Read the model definition and answer for the solid it produces. Units are mm, in the model's axes. A direction names the side the tool comes from. Give positions to 0.01 mm unless a question says otherwise; leave off trailing zeros. Loops run counter-clockwise (first coordinate to the right, second up) from the corner with the lowest first, then second, coordinate; pieces in that order, holes last. Notation, with made-up numbers: (48, 46.5) - (69, 46.5) arc R14 ccw to (69, 54.5) - close; hole circle Ø2 at (-29, 71.5). An arc over 180 degrees is marked (long way). Write item = value, one per line.
```python
from build123d import *

# Parameters (mm, degrees)
BOSS_EXTRUDE1_DEPTH = 1.524


with BuildPart() as part:
    # Sketch1 → Boss-Extrude1 (new body)
    with BuildSketch(Plane.XY):
        with BuildLine():
            Line((25.899875794, 0), (25.899875794, -1.524))
            Line((25.899875794, -1.524), (22.32048354, -1.524))
            ThreePointArc((22.32048354, -1.524), (22.394704152, -2.448389179), (22.608367924, -3.350803633))
            ThreePointArc((22.608367924, -3.350803633), (24.775682693, -15.358642742), (23.925034543, -27.530818024))
            ThreePointArc((23.925034543, -27.530818024), (24.269313487, -29.941018013), (26.694765546, -30.152617376))
            ThreePointArc((26.694765546, -30.152617376), (43.800025443, -37.203050355), (61.874254559, -41.155361478))
            ThreePointArc((61.874254559, -41.155361478), (63.35881503, -45.79590736), (63.615238945, -50.661380887))
            ThreePointArc((63.615238945, -50.661380887), (65.284550388, -52.552507853), (66.8346767, -50.562515312))
            ThreePointArc((66.8346767, -50.562515312), (66.086863923, -45.883082095), (65.762862434, -41.155361478))
            ThreePointArc((65.762862434, -41.155361478), (66.787088001, -38.530646728), (65.033651376, -36.325283826))
            ThreePointArc((65.033651376, -36.325283826), (63.508505747, -35.385780492), (62.493571354, -33.909757498))
            ThreePointArc((62.493571354, -33.909757498), (60.142882659, -34.378985159), (58.743656643, -36.325283826))
            ThreePointArc((58.743656643, -36.325283826), (57.410289813, -36.601347141), (56.250770366, -35.887489516))
            ThreePointArc((56.250770366, -35.887489516), (55.059942052, -35.328446838), (53.862175702, -34.784427942))
            ThreePointArc((53.862175702, -34.784427942), (53.387744375, -32.845536507), (52.235990682, -31.215245578))
            ThreePointArc((52.235990682, -31.215245578), (52.379437809, -32.619080701), (52.025456966, -33.985106943))
            ThreePointArc((52.025456966, -33.985106943), (49.256787636, -32.858021413), (46.457035721, -31.810528756))
            ThreePointArc((46.457035721, -31.810528756), (45.520333016, -29.932577753), (43.969177054, -28.519061884))
            ThreePointArc((43.969177054, -28.519061884), (44.348322504, -29.737128844), (43.969177054, -30.955195804))
            ThreePointArc((43.969177054, -30.955195804), (40.682262853, -29.930853217), (37.363411838, -29.015260162))
            ThreePointArc((37.363411838, -29.015260162), (36.338596802, -27.1840345), (34.737637182, -25.82736152))
            ThreePointArc((34.737637182, -25.82736152), (35.485911293, -27.135318264), (35.76553834, -28.616018674))
            ThreePointArc((35.76553834, -28.616018674), (32.102551283, -27.80064259), (28.412668556, -27.117211688))
            ThreePointArc((28.412668556, -27.117211688), (27.08385139, -27.186040378), (26.694765546, -25.913599945))
            ThreePointArc((26.694765546, -25.913599945), (26.802310466, -25.249830728), (26.908212993, -24.585797492))
            ThreePointArc((26.908212993, -24.585797492), (27.859098363, -23.097961687), (29.420120996, -22.272706147))
            ThreePointArc((29.420120996, -22.272706147), (28.583123123, -21.317792963), (27.500905932, -20.653541067))
            ThreePointArc((27.500905932, -20.653541067), (27.824154163, -18.325383322), (28.127257878, -15.994517379))
            ThreePointArc((28.127257878, -15.994517379), (28.758910246, -15.256602171), (29.730007897, -15.234855434))
            ThreePointArc((29.730007897, -15.234855434), (28.962069061, -13.633439137), (28.611030242, -11.892452072))
            ThreePointArc((28.611030242, -11.892452072), (28.885875625, -9.28370644), (29.135532328, -6.672429877))
            ThreePointArc((29.135532328, -6.672429877), (30.079064964, -6.355518981), (31.070294126, -6.44580243))
            ThreePointArc((31.070294126, -6.44580243), (29.85894962, -5.077426559), (29.420124937, -3.303380072))
            ThreePointArc((29.420124937, -3.303380072), (29.431447758, -3.003641616), (29.466206898, -2.705710163))
            ThreePointArc((29.466206898, -2.705710163), (29.538300485, -1.73398118), (29.606910148, -0.762))
            ThreePointArc((29.606910148, -0.762), (29.438405233, 0.690848146), (28.412668556, 1.733453494))
            ThreePointArc((28.412668556, 1.733453494), (26.035003808, 1.415915884), (23.657339059, 1.733453494))
            ThreePointArc((23.657339059, 1.733453494), (22.643555103, 1.133068669), (22.32048354, 0))
            Line((22.32048354, 0), (25.899875794, 0))
        make_face()
    extrude(amount=BOSS_EXTRUDE1_DEPTH)


solid = part.part
```
1) A tool of negligible diameter and unlimited length cuts with its end or side. For faces 1 (the face through (30.065, -6.357, 0.751)), 2 (the face through (24, 0, 1)), 3 (the face through (28.97, -13.66, 0.75)), 4 (the face through (40.729, -29.944, 0.751)), from which of +Z, -Z, +X, -X, +Y, -Y can it reach the whole face along a straight path? Write none if from no direction.
Output:
face_1 = +Z, -Z
face_2 = +Z, -Z, -X
face_3 = +Z, -Z, +X
face_4 = +Z, -Z, +Y
2) A cutting plane is placed at A-A on x = 50.5. Determine the outline of the cut face in (y, z), then the cut area to 3 significant figures.
Output:
outline = (-39.06, 0) - (-33.35, 0) - (-33.35, 1.52) - (-39.06, 1.52) - close
area = 8.70 mm²
3) Find the intervals of material crossed by probe 1 along X at (y, z) = (-33.5, 1.3); probe 2 along Y at (x, z) = (35, 0.5); probe 3 along Y at (x, z) = (33, 0.6), in increasing order.
Output:
probe_1 = 33.77 to 50.86, 52.21 to 53.64
probe_2 = -34.02 to -28.43, -26.18 to -25.99
probe_3 = -33.16 to -27.99
4) The mould has two halves that part along Y. Classify faces 5 (the face through (36.36, -27.21, 0.75)), 6 (the face through (44.5, -29.3, 1.524)), 7 (the face through (52.38, -32.6, 0.75)): pulls with the +Y half, pulls with the -Y half, needs draft (parallel to the pull), parting line crosses it, or undercut.
Output:
face_5 = pulls with the +Y half
face_6 = needs draft
face_7 = undercut
5) Each of these flat-tipped pins is pushed along its axis until it touches: P1, Ø0.5, axis at y = -0.5, z = 0.5, coming from the -X side; P2, Ø12, axis at x = 47, y = -45, coming from the -Z side. Where does it stop, or does it pass through?
Output:
P1 = 25.9
P2 = through
6) A cutting plane is placed at B-B on y = -4. Determine the outline of the cut face in (x, z), then the cut area to 3 significant figures.
Output:
outline = (22.81, 0) - (29.49, 0) - (29.49, 1.52) - (22.81, 1.52) - close
area = 10.2 mm²
